from build123d import *

# Parameters (mm, degrees)
SKETCH2_R           = 7.5
BOSS_EXTRUDE1_DEPTH = 58
CUT_EXTRUDE1_DEPTH  = 107.60206377
DRAFT2_ANGLE        = 45
SKETCH6_R           = 7
CUT_EXTRUDE6_DEPTH  = 107.60206377
CHAMFER9_START      = 91.570328164
CHAMFER9_OUTLINE_W  = 15
CHAMFER9_OUTLINE_H  = 42
CHAMFER9_DEPTH      = 7.429671836
CHAMFER10_START     = -58
CHAMFER10_OUTLINE_W = 15
CHAMFER10_OUTLINE_H = 42
CHAMFER10_DEPTH     = 7.441865145


with BuildPart() as part:
    # Sketch2 → Boss-Extrude1 (new body)
    with BuildSketch(Plane(origin=(0, 0, 0), x_dir=(0, 0, -1), z_dir=(1, 0, 0))):
        with BuildLine():
            Line((0, 0), (0, 24))
            ThreePointArc((0, 24), (16.66060556, 35.82575695), (36.66060556, 40))
            Line((36.66060556, 40), (65, 40))
            Line((65, 40), (80, 31.339745962))
            Line((80, 31.339745962), (80, 8.660254038))
            Line((80, 8.660254038), (65, 0))
            Line((65, 0), (0, 0))
        make_face()
        with Locations(Location((31, 19, 0), (0, 0, 180))):
            Circle(SKETCH2_R, mode=Mode.SUBTRACT)
    extrude(amount=BOSS_EXTRUDE1_DEPTH)

    # Sketch4 → Cut-Extrude1 (cut, through all)
    with BuildSketch(Plane.XZ):
        Polygon((8, 0), (50, 0), (50, -16), (44, -16), (44, -54), (14, -54), (14, -16), (8, -16), align=None)
    extrude(amount=-CUT_EXTRUDE1_DEPTH, mode=Mode.SUBTRACT)

    # Draft2
    draft2_faces = [part.faces().sort_by_distance(p)[0] for p in [
        (29, 4.330127019, -72.5),
        (29, 35.669872981, -72.5),
    ]]
    draft(draft2_faces, Plane(origin=(58, 8.660254038, -80), x_dir=(-1, 0, 0), z_dir=(0, 0, -1)), DRAFT2_ANGLE)

    # Sketch6 → Cut-Extrude6 (cut, through all)
    with BuildSketch(Plane(origin=(0, 0, -80), x_dir=(-1, 0, 0), z_dir=(0, 0, -1))):
        with Locations((-29, 20)):
            Circle(SKETCH6_R)
    extrude(amount=-CUT_EXTRUDE6_DEPTH, mode=Mode.SUBTRACT)

    # Chamfer9: read off the stored shape, not the designer's step
    # Chamfer9 outline → Chamfer9 (cut)
    with BuildSketch(Plane(origin=(0, 0, 0), x_dir=(0.707106781186548, 0, 0.707106781186547), z_dir=(0.707106781186547, 0, -0.707106781186548)).offset(CHAMFER9_START)):
        with Locations((-15.5, -20)):
            Rectangle(CHAMFER9_OUTLINE_W, CHAMFER9_OUTLINE_H)
    extrude(amount=CHAMFER9_DEPTH, mode=Mode.SUBTRACT)

    # Chamfer10: read off the stored shape, not the designer's step
    # Chamfer10 outline → Chamfer10 (cut)
    with BuildSketch(Plane(origin=(0, 0, 0), x_dir=(0.707106781186548, 0, -0.707106781186547), z_dir=(0.707106781186547, 0, 0.707106781186548)).offset(CHAMFER10_START)):
        with Locations((56.5, 20)):
            Rectangle(CHAMFER10_OUTLINE_W, CHAMFER10_OUTLINE_H)
    extrude(amount=CHAMFER10_DEPTH, mode=Mode.SUBTRACT)


solid = part.part
Read the model definition and answer for the solid it produces. Units are mm, in the model's axes. A direction names the side the tool comes from. Give positions to 0.01 mm unless a question says otherwise; leave off trailing zeros. Write each loop counter-clockwise with the first axis right and the second up, starting at its lowest first coordinate (ties: lowest second). Pieces come first, ordered by that corner, then holes. Notation, with made-up numbers: (61.25, 55.5) - (116.25, 55.5) arc R29 cw to (116.25, 87.5) - close; hole circle Ø3 at (65, -20.75). An arc over 180 degrees is marked (long way). Use CSV: the item, a comma, the result in double quotes. Start each with the question number.
(1) Consider line 1 along X through (y, z) = (23, -17.5); line 2 along Z through (x, y) = (11, 19); line 3 along Y through (x, z) = (29, -69). Determine where each line is inside the solid, lowest interval first.
(2) Determine the mould class of faces 3 (the flat face through (0, 20, -44)), 4 (the cylindrical face through (6.9, 13.9, -36.5)), 5 (the flat face through (47, 18, -16)) for opening direction X: +X half, -X half, draft (parallel to the pull), parting line (faces both ways), or undercut.
(3) Find section D-D (z = -31). Give the vertices of the cut face in (x, y).
(4) Find section A-A (z = -47). Give the vertices of the cut face in (x, y).
(5) Given P1, Ø8, axis at x = 22.5, y = 4.5, coming from the -Z side; P2, Ø5, axis at x = 11.5, y = 15, coming from the +Z side, each flat-ended and moving along its own axis, determine where each tip first touches the part or whether it passes through.
(6) Find section C-C (y = 10). Give the vertices of the cut face in (x, z), plus the area to 3 significant figures.
(7) Find section B-B (x = 29). Give the vertices of the cut face in (y, z).
(8) For faces 1 (the flat face through (44, 20, -39)), 2 (the flat face through (4.2, 20.3, -75.7)), determine the directions among +Z, -Z, +X, -X, +Y, -Y from which every point of the face is accessible in a straight line to the end or side of a thin tool.
Findings below:
1,line 1,"0 to 14, 44 to 58"
1,line 2,"-80 to -38.5, -23.5 to -16"
1,line 3,"0 to 13, 27 to 40"
2,face 3,"-X half"
2,face 4,"draft"
2,face 5,"undercut"
3,outline,"(0, 0) - (14, 0) - (14, 11.5) - (0, 11.5) - close; (0, 26.5) - (14, 26.5) - (14, 39.68) - (0, 39.68) - close; (44, 0) - (58, 0) - (58, 11.5) - (44, 11.5) - close; (44, 26.5) - (58, 26.5) - (58, 39.68) - (44, 39.68) - close"
4,outline,"(0, 0) - (14, 0) - (14, 40) - (0, 40) - close; (44, 0) - (58, 0) - (58, 40) - (44, 40) - close"
5,P1,"z = -79.84"
5,P2,"z = -16"
6,outline,"(0, -71.5) - (8.5, -80) - (49.5, -80) - (58, -71.5) - (58, 0) - (50, 0) - (50, -16) - (44, -16) - (44, -54) - (14, -54) - (14, -16) - (8, -16) - (8, 0) - (0, 0) - close"
6,area,"2,760 mm2"
7,outline,"(0, -71.34) - (8.66, -80) - (13, -80) - (13, -54) - (0, -54) - close; (27, -80) - (31.34, -80) - (40, -71.34) - (40, -54) - (27, -54) - close"
8,face 1,"+Z, +Y, -Y"
8,face 2,"-Z, -X, +Y, -Y"
